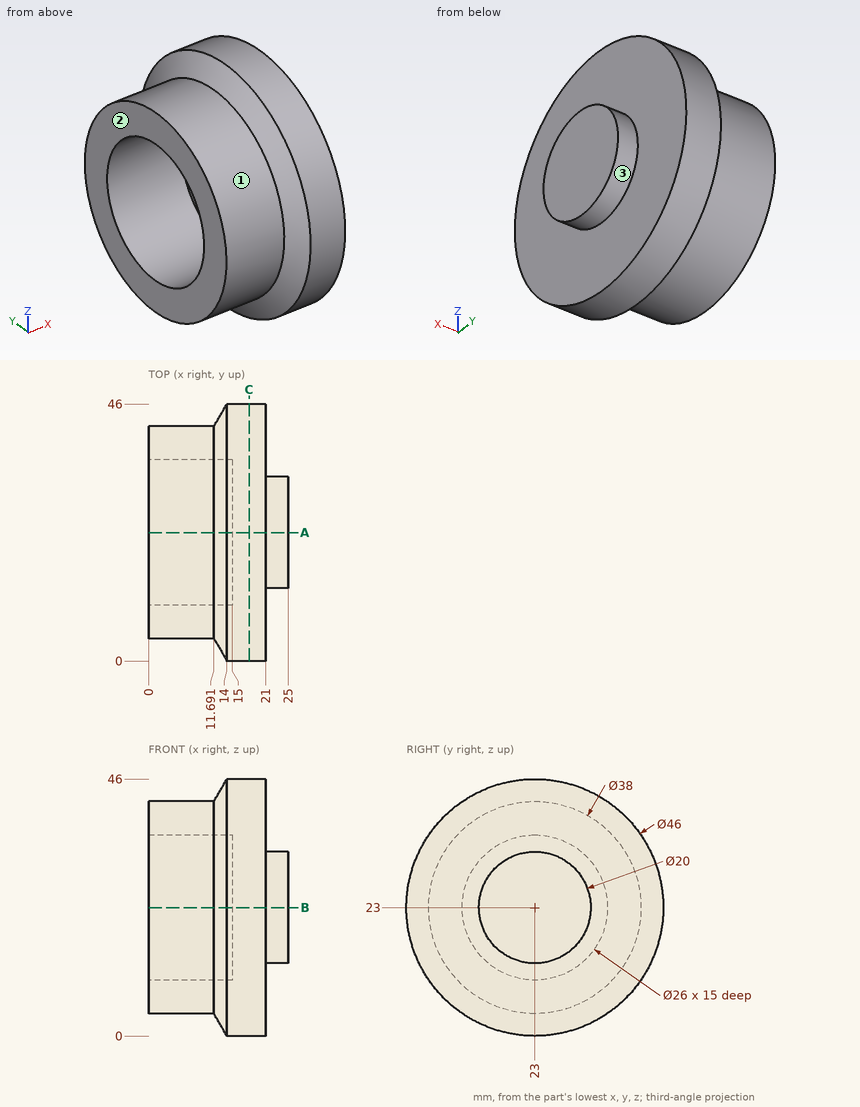
Study the drawing (mm; zero at the part's minimum x, y, z) and answer. A direction names the side the tool comes from. Round coordinates to 2 decimals unless told otherwise and drop trailing zeros. Loops run counter-clockwise (first coordinate to the right, second up) from the corner with the lowest first, then second, coordinate; pieces in that order, holes last. Notation, with made-up numbers: (85, 83.5) -> (110, 83.5) arc R16 cw to (110, 96.5) -> close; hole circle Ø10 at (16.25, -29). An arc over 180 degrees is marked (long way). Use one line per item in the form item = value.
1. A tool of negligible diameter and unlimited length cuts with its end or side. For the marked faces 1, 2 and 3, from which of +Z, -Z, +X, -X, +Y, -Y can it reach the whole face along a straight path? Write none if from no direction.
Answer key:
face_1 = -X
face_2 = +Z, -Z, -X, +Y, -Y
face_3 = +X
2. Find the intervals of material crossed by probe 1 along Y at (x, z) = (8, 23); probe 2 along Z at (x, y) = (1.75, 33) (1 decimal); probe 3 along X at (y, z) = (27, 24), in increasing order. Write a range as [from, to].
Answer key:
probe_1 = [4, 10], [36, 42]
probe_2 = [6.8, 14.7], [31.3, 39.2]
probe_3 = [15, 25]
3. The part is cut by section A-A on y = 23. Determine the outline of the cut face in (x, z).
Answer key:
outline = (0, 4) -> (11.69, 4) -> (14, 0) -> (21, 0) -> (21, 13) -> (25, 13) -> (25, 33) -> (21, 33) -> (21, 46) -> (14, 46) -> (11.69, 42) -> (0, 42) -> (0, 36) -> (15, 36) -> (15, 10) -> (0, 10) -> close
4. Flat-ended cylindrical pins translate along their axes: pin 1 Ø4 at (x, y) = (14, 11.5) entering from +Z; pin 2 Ø6 at (x, y) = (20, 37.5) entering from +Z; pin 3 Ø3 at (x, y) = (19.5, 19.5) entering from +Z. Find the tip coordinate at first contact, or state that the pin passes through.
Answer key:
pin_1 = 43.95
pin_2 = 42.92
pin_3 = 45.91
5. The part is cut by section C-C on x = 18. Determine the outline of the cut face in (y, z), and give its area (3 significant figures).
Answer key:
outline = circle Ø46 at (23, 23)
area = 1,660 mm²
